Input: part model. Units: mm. Frame: model coordinates. Face numbers are marked on the shaded views. Round coordinates to 2 decimals unless told otherwise and drop trailing zeros. Loops run counter-clockwise (first coordinate to the right, second up) from the corner with the lowest first, then second, coordinate; pieces in that order, holes last. Notation, with made-up numbers: (31.25, -8) -> (81.25, -8) arc R22 cw to (81.25, 5) -> close; hole circle Ø7 at (60, 31.5). An arc over 180 degrees is marked (long way). Answer in a Markdown table with one row per item. Add a question column.
Q1. Section A-A, the plane z = 5. Output: boundary loops of the cut face in (x, y), and give its area (3 significant figures).
Q2. Section B-B, the plane x = 5. Output: boundary loops of the cut face in (y, z), and give its area (3 significant figures).
Q3. Ray query, L1, parallel to Z at x = 5, y = 5.5; L2, parallel to Z at x = 4, y = 9.25; L3, parallel to X at y = 3.75, z = 5. Return the intervals inside material, ascending. Write a range as from..to.
Q4. Mould query, pull axis Z, two halves, no side actions, for the marked faces 1, 2, 3 and 4. Classes: pulls with the +Z half, pulls with the -Z half, needs draft (parallel to the pull), parting line crosses it, or undercut.
Q5. Section C-C, the plane y = 7.5. Output: boundary loops of the cut face in (x, z), and give its area (3 significant figures).
Autodesk Inventor part; units mm, degrees
ref_plane "YZ Plane" through (0, 0, 0) normal (1, 0, 0) x (0, 1, 0)
ref_plane "XZ Plane" through (0, 0, 0) normal (0, 1, 0) x (-1, 0, 0)
ref_plane "XY Plane" through (0, 0, 0) normal (0, 0, 1) x (1, 0, 0)
sketch "スケッチ1" plane through (0, 0, 0) normal (0, 0, 1) x (1, 0, 0)
  line L0 (0, 0) -> (10, 0)
  line L1 (10, 0) -> (10, 10)
  line L2 (10, 10) -> (0, 10)
  line L3 (0, 10) -> (0, 0)
  dimension "d0" = 10
  dimension "d1" = 10
extrude "押し出し1" add sketch "スケッチ1" along normal blind 60
sketch "スケッチ2" plane through (0, 10, 0) normal (0, 1, 0) x (1, 0, 0)
  line L0 (0, 0) -> (0, -60)
  line L1 (10, 0) -> (0, 0)
  point P0 (5, -5)
  dimension "d4" = 5
  dimension "d5" = 5
hole "穴1" at (5, 10, 5) direction (0, -1, 0) diameter 6 end through all
sketch "スケッチ3" plane through (0, 10, 0) normal (0, 1, 0) x (1, 0, 0)
  line L0 (0, 0) -> (0, -60)
  line L1 (10, 0) -> (0, 0)
  point P0 (5, -25)
  dimension "d13" = 5
  dimension "d14" = 25
hole "穴2" at (5, 10, 25) direction (0, -1, 0) diameter 6 end through all
properties part number "アーム10×10×60"
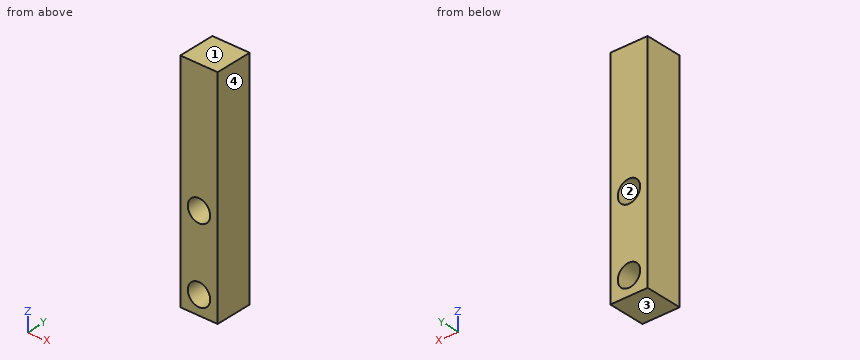
Answer block:
| question | item | result |
|---|---|---|
| 1 | outline | (0, 0) -> (2, 0) -> (2, 10) -> (0, 10) -> close; (8, 0) -> (10, 0) -> (10, 10) -> (8, 10) -> close |
| 1 | area | 40.0 mm^2 |
| 2 | outline | (0, 0) -> (10, 0) -> (10, 2) -> (0, 2) -> close; (0, 8) -> (10, 8) -> (10, 22) -> (0, 22) -> close; (0, 28) -> (10, 28) -> (10, 60) -> (0, 60) -> close |
| 2 | area | 480 mm^2 |
| 3 | L1 | 0..2, 8..22, 28..60 |
| 3 | L2 | 0..2.17, 7.83..22.17, 27.83..60 |
| 3 | L3 | 0..2, 8..10 |
| 4 | face 1 | pulls with the +Z half |
| 4 | face 2 | undercut |
| 4 | face 3 | pulls with the -Z half |
| 4 | face 4 | needs draft |
| 5 | outline | (0, 0) -> (10, 0) -> (10, 60) -> (0, 60) -> close; hole circle Ø6 at (5, 5); hole circle Ø6 at (5, 25) |
| 5 | area | 543 mm^2 |
